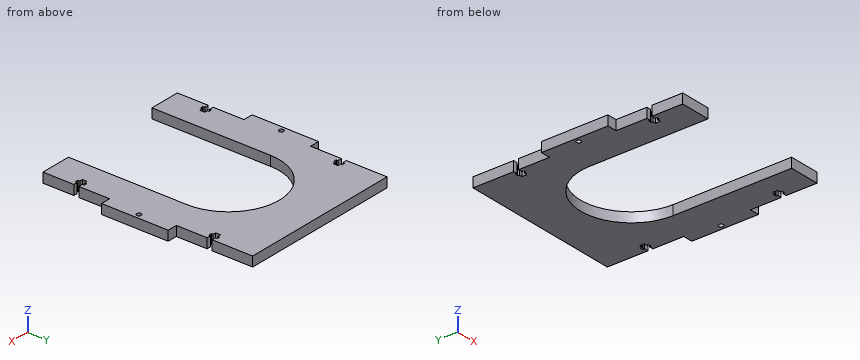
```python
from build123d import *

# Parameters (mm, degrees)
SKETCH1_R           = 1.5
BOSS_EXTRUDE1_DEPTH = 6.35


with BuildPart() as part:
    # Sketch1 → Boss-Extrude1 (new body)
    with BuildSketch(Plane.XY):
        with BuildLine():
            Line((6.35, 6.35), (6.35, -20.066666667))
            Line((6.35, -20.066666667), (9, -20.066666667))
            Line((9, -20.066666667), (9, -18.916666667))
            Line((9, -18.916666667), (11, -18.916666667))
            Line((11, -18.916666667), (11, -20.066666667))
            Line((11, -20.066666667), (13, -20.066666667))
            Line((13, -20.066666667), (13, -23.266666667))
            Line((13, -23.266666667), (11, -23.266666667))
            Line((11, -23.266666667), (11, -24.416666667))
            Line((11, -24.416666667), (9, -24.416666667))
            Line((9, -24.416666667), (9, -23.266666667))
            Line((9, -23.266666667), (6.35, -23.266666667))
            Line((6.35, -23.266666667), (6.35, -43.333333333))
            Line((6.35, -43.333333333), (0, -43.333333333))
            Line((0, -43.333333333), (0, -86.666666667))
            Line((0, -86.666666667), (6.35, -86.666666667))
            Line((6.35, -86.666666667), (6.35, -106.733333333))
            Line((6.35, -106.733333333), (9, -106.733333333))
            Line((9, -106.733333333), (9, -105.583333333))
            Line((9, -105.583333333), (11, -105.583333333))
            Line((11, -105.583333333), (11, -106.733333333))
            Line((11, -106.733333333), (13, -106.733333333))
            Line((13, -106.733333333), (13, -109.933333333))
            Line((13, -109.933333333), (11, -109.933333333))
            Line((11, -109.933333333), (11, -111.083333333))
            Line((11, -111.083333333), (9, -111.083333333))
            Line((9, -111.083333333), (9, -109.933333333))
            Line((9, -109.933333333), (6.35, -109.933333333))
            Line((6.35, -109.933333333), (6.35, -130))
            Line((6.35, -130), (26.35, -130))
            Line((26.35, -130), (26.35, -53))
            ThreePointArc((26.35, -53), (59.35, -20), (92.35, -53))
            Line((92.35, -53), (92.35, -130))
            Line((92.35, -130), (112.35, -130))
            Line((112.35, -130), (112.35, -109.933333333))
            Line((112.35, -109.933333333), (109.7, -109.933333333))
            Line((109.7, -109.933333333), (109.7, -111.083333333))
            Line((109.7, -111.083333333), (107.7, -111.083333333))
            Line((107.7, -111.083333333), (107.7, -109.933333333))
            Line((107.7, -109.933333333), (105.7, -109.933333333))
            Line((105.7, -109.933333333), (105.7, -106.733333333))
            Line((105.7, -106.733333333), (107.7, -106.733333333))
            Line((107.7, -106.733333333), (107.7, -105.583333333))
            Line((107.7, -105.583333333), (109.7, -105.583333333))
            Line((109.7, -105.583333333), (109.7, -106.733333333))
            Line((109.7, -106.733333333), (112.35, -106.733333333))
            Line((112.35, -106.733333333), (112.35, -86.666666667))
            Line((112.35, -86.666666667), (118.7, -86.666666667))
            Line((118.7, -86.666666667), (118.7, -43.333333333))
            Line((118.7, -43.333333333), (112.35, -43.333333333))
            Line((112.35, -43.333333333), (112.35, -23.266666667))
            Line((112.35, -23.266666667), (109.7, -23.266666667))
            Line((109.7, -23.266666667), (109.7, -24.416666667))
            Line((109.7, -24.416666667), (107.7, -24.416666667))
            Line((107.7, -24.416666667), (107.7, -23.266666667))
            Line((107.7, -23.266666667), (105.7, -23.266666667))
            Line((105.7, -23.266666667), (105.7, -20.066666667))
            Line((105.7, -20.066666667), (107.7, -20.066666667))
            Line((107.7, -20.066666667), (107.7, -18.916666667))
            Line((107.7, -18.916666667), (109.7, -18.916666667))
            Line((109.7, -18.916666667), (109.7, -20.066666667))
            Line((109.7, -20.066666667), (112.35, -20.066666667))
            Line((112.35, -20.066666667), (112.35, 6.35))
            Line((112.35, 6.35), (6.35, 6.35))
        make_face()
        with Locations((3.175, -65)):
            Circle(SKETCH1_R, mode=Mode.SUBTRACT)
        with Locations((115.525, -65)):
            Circle(SKETCH1_R, mode=Mode.SUBTRACT)
    extrude(amount=BOSS_EXTRUDE1_DEPTH)


solid = part.part
```
Input: part model. Units: mm. Frame: model coordinates. Give positions to 0.01 mm unless a question says otherwise; leave off trailing zeros. Order: outer loops, then holes, each group sorted by start corner. A loop starts at its lowest first (then second) coordinate and runs counter-clockwise, first axis right, second up. Notation, with made-up numbers: M 71.25,10.5 L 98.25,10.5 A22 ccw 98.25,47.5 Z; hole C 87,-22 d9. An arc over 180 degrees is marked long. Return JSON: item names as keys, results as strings.
1) Section query D-D on z = 2. Count the separate pieces of the cut face and the enclosed holes in it, and give its area (3 significant figures).
Taken from the geometry:
{"separate pieces": "1", "enclosed holes": "2", "area": "8,090 mm2"}
2) Section query A-A on y = -90.5. Output: boundary loops of the cut face in (x, z), and give its area (3 significant figures).
Taken from the geometry:
{"outline": "M 6.35,0 L 26.35,0 L 26.35,6.35 L 6.35,6.35 Z; M 92.35,0 L 112.35,0 L 112.35,6.35 L 92.35,6.35 Z", "area": "254 mm2"}
3) Section query C-C on x = 59.35. Output: boundary loops of the cut face in (y, z).
Taken from the geometry:
{"outline": "M -20,0 L 6.35,0 L 6.35,6.35 L -20,6.35 Z"}
4) Contact query for flat-ended pins moving along their axis: pin 1 (3 mm diameter, centred on y = -94, z = 5, fed in from -X); pin 2 (3 mm diameter, centred on x = 59.5, z = 5.5, fed in from -Y); pin 3 (0.9 mm diameter, centred on y = -106, z = 2, fed in from +X). Output: stop coordinate, or through.
Taken from the geometry:
{"pin 1": "stops at x = 6.35", "pin 2": "stops at y = -20.04", "pin 3": "stops at x = 112.35"}
5) Line query: L1, parallel to X at y = -65, z = 3 (3 decimals); L2, parallel to X at y = -78, z = 5.75; L3, parallel to X at y = -119, z = 1.25. Output: solid intervals per line, ascending. Write a range as [from, to].
Taken from the geometry:
{"L1": "x = [0, 1.675], [4.675, 26.35], [92.35, 114.025], [117.025, 118.7]", "L2": "x = [0, 26.35], [92.35, 118.7]", "L3": "x = [6.35, 26.35], [92.35, 112.35]"}
6) Section query B-B on y = -71.5. Output: boundary loops of the cut face in (x, z), and give its area (3 significant figures).
Taken from the geometry:
{"outline": "M 0,0 L 26.35,0 L 26.35,6.35 L 0,6.35 Z; M 92.35,0 L 118.7,0 L 118.7,6.35 L 92.35,6.35 Z", "area": "335 mm2"}
